CAD build for the part. Positions are in the model's coordinates, mm. Face numbers are marked on the shaded views. Round coordinates to 2 decimals unless told otherwise and drop trailing zeros. Order: outer loops, then holes, each group sorted by start corner. A loop starts at its lowest first (then second) coordinate and runs counter-clockwise, first axis right, second up.
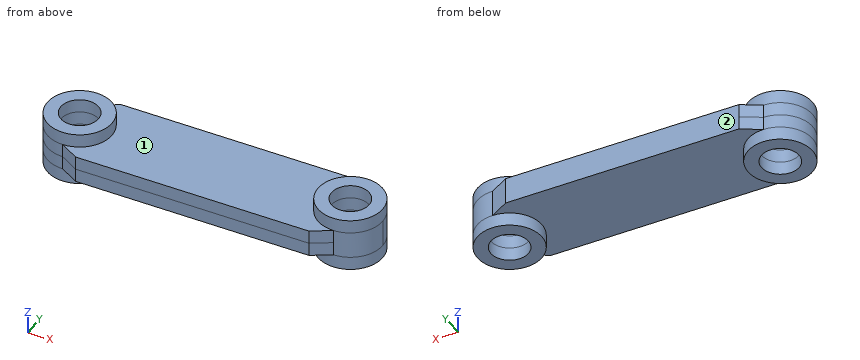
```python
from build123d import *

# Parameters (mm, degrees)
SKETCH1_R           = 6
SKETCH1_R_2         = 3.5
BOSS_EXTRUDE1_DEPTH = 2.5
SKETCH4_R           = 6
SKETCH4_R_2         = 3.5
BOSS_EXTRUDE2_DEPTH = 5


with BuildPart() as part:
    # Sketch1 → Boss-Extrude1 (new, symmetric)
    # profile 1 of 3: a face of its own
    with BuildSketch(Plane.XY):
        with BuildLine():
            Line((3.464101615, 8), (0, 6))
            ThreePointArc((0, 6), (4.242640687, 4.242640687), (6, 0))
            ThreePointArc((6, 0), (4.242640687, -4.242640687), (0, -6))
            Line((0, -6), (3.464101615, -8))
            Line((3.464101615, -8), (46.535898385, -8))
            Line((46.535898385, -8), (50, -6))
            ThreePointArc((50, -6), (44, 0), (50, 6))
            Line((50, 6), (46.535898385, 8))
            Line((46.535898385, 8), (3.464101615, 8))
        make_face()
    # profile 2 of 3: a face of its own
    with BuildSketch(Plane.XY):
        Circle(SKETCH1_R)
        Circle(SKETCH1_R_2, mode=Mode.SUBTRACT)
    # profile 3 of 3: a face of its own
    with BuildSketch(Plane.XY):
        with Locations((50, 0)):
            Circle(SKETCH1_R)
        with Locations((50, 0)):
            Circle(SKETCH1_R_2, mode=Mode.SUBTRACT)
    extrude(amount=BOSS_EXTRUDE1_DEPTH, both=True)

    # Sketch4 → Boss-Extrude2 (add, symmetric)
    # profile 1 of 2: a face of its own
    with BuildSketch(Plane.XY):
        Circle(SKETCH4_R)
        Circle(SKETCH4_R_2, mode=Mode.SUBTRACT)
    # profile 2 of 2: a face of its own
    with BuildSketch(Plane.XY):
        with Locations((50, 0)):
            Circle(SKETCH4_R)
        with Locations((50, 0)):
            Circle(SKETCH4_R_2, mode=Mode.SUBTRACT)
    extrude(amount=BOSS_EXTRUDE2_DEPTH, both=True)


solid = part.part
```
1. Cut at C-C, the plane y = 2. Write the cut outline in (x, z), and give its area (3 significant figures).
2. Mould opens along X. For the marked faces 1 and 2 say: released by +X, released by -X, zero draft, split by the parting line, or undercut.
3. Cut at B-B, the plane z = -4. Write the cut outline in (x, y), and give its area (3 significant figures).
4. Drill centre lines: line 1 (Y direction, x = 0, z = -3.2); line 2 (X direction, y = -0.75, z = 3.75); line 3 (X direction, y = 2.75, z = 4.5). Where is each one in solid material? Low to high.
5. Pin check, flat tips, straight feed: P1, Ø3, axis at x = 35.5, y = -1.5, coming from the +Z side; P2, Ø5.5, axis at x = 50, y = 0, coming from the -Z side; P3, Ø4, axis at x = 8, y = -2, coming from the -Z side; P4, Ø1, axis at y = 5.5, z = -2, coming from the -X side. Stop position of each tip, or through.
6. Cut at D-D, the plane y = -4.25. Write the cut outline in (x, z), and give its area (3 significant figures).
7. Cut at A-A, the plane x = 51.5. Write the cut outline in (y, z).
Outcome:
1. outline: (-5.66, -5) - (-2.87, -5) - (-2.87, 5) - (-5.66, 5) - close; (2.87, -5) - (5.66, -5) - (5.66, -2.5) - (44.34, -2.5) - (44.34, -5) - (47.13, -5) - (47.13, 5) - (44.34, 5) - (44.34, 2.5) - (5.66, 2.5) - (5.66, 5) - (2.87, 5) - close; (52.87, -5) - (55.66, -5) - (55.66, 5) - (52.87, 5) - close
1. area: 305 mm2
2. face 1: undercut
2. face 2: zero draft
3. outline: circle Ø12 at (0, 0); circle Ø12 at (50, 0); hole circle Ø7 at (0, 0); hole circle Ø7 at (50, 0)
3. area: 149 mm2
4. line 1: y = -6 to -3.5, 3.5 to 6
4. line 2: x = -5.95 to -3.42, 3.42 to 5.95, 44.05 to 46.58, 53.42 to 55.95
4. line 3: x = -5.33 to -2.17, 2.17 to 5.33, 44.67 to 47.83, 52.17 to 55.33
5. P1: stops at z = 2.5
5. P2: passes through
5. P3: stops at z = -2.5
5. P4: stops at x = -3.32
6. outline: (-4.24, -5) - (4.24, -5) - (4.24, -2.5) - (45.76, -2.5) - (45.76, -5) - (54.24, -5) - (54.24, 5) - (45.76, 5) - (45.76, 2.5) - (4.24, 2.5) - (4.24, 5) - (-4.24, 5) - close
6. area: 377 mm2
7. outline: (-5.81, -5) - (-3.16, -5) - (-3.16, 5) - (-5.81, 5) - close; (3.16, -5) - (5.81, -5) - (5.81, 5) - (3.16, 5) - close
